from build123d import *

# Parameters (mm, degrees)
BOSS_EXTRUDE1_DEPTH      = 50
BOSS_EXTRUDE1_DEPTH_BACK = 50
SKETCH2_W                = 10
SKETCH2_H                = 3
SKETCH3_W                = 5
SKETCH3_H                = 3
SKETCH5_R                = 1.5
CUT_EXTRUDE2_DEPTH       = 3


with BuildPart() as part:
    # Sketch2 → Boss-Extrude1 (new, two sides: drawn at the far end of the back side and taken through both)
    with BuildSketch(Plane.XY.offset(-BOSS_EXTRUDE1_DEPTH_BACK)):
        with Locations((-5, -1)):
            Rectangle(SKETCH2_W, SKETCH2_H)
    extrude(amount=BOSS_EXTRUDE1_DEPTH + BOSS_EXTRUDE1_DEPTH_BACK)

    # Sketch3 → Revolve1 (revolve)
    with BuildSketch(Plane.XY.offset(50)):
        with Locations((-2.5, -1)):
            Rectangle(SKETCH3_W, SKETCH3_H)
    revolve1 = revolve(axis=Axis((-5, 0.5, 50), (0, -1, 0)))

    # Mirror1: Revolve1 across plane
    add(revolve1.mirror(Plane.XY))

    # Sketch5 → Cut-Extrude2 (cut)
    with BuildSketch(Plane(origin=(0, -2.5, 0), x_dir=(-1, 0, 0), z_dir=(0, -1, 0))):
        with Locations(Location((5, -50, 0), (0, 0, 180))):
            Circle(SKETCH5_R)
    cut_extrude2 = extrude(amount=-CUT_EXTRUDE2_DEPTH, mode=Mode.SUBTRACT)

    # Mirror2: Cut-Extrude2 across plane
    add(cut_extrude2.mirror(Plane.XY), mode=Mode.SUBTRACT)


solid = part.part
Input: part model. Units: mm. Frame: model coordinates. Round coordinates to 2 decimals unless told otherwise and drop trailing zeros. Write each loop counter-clockwise with the first axis right and the second up, starting at its lowest first coordinate (ties: lowest second). Pieces come first, ordered by that corner, then holes.
1) Contact query for a flat-ended pin moving along its axis: P1, Ø1, axis at x = -8.5, y = -1.5, coming from the +Z side. Output: stop coordinate, or through.
2) Ray query, L1, parallel to Z at x = -5, y = -0.65; L2, parallel to X at y = -0.55, z = -50; L3, parallel to Z at x = -4.5, y = -2.25. Return the intervals inside material, ascending.
3) Cut plane B-B (y = -2). Return the cut outline in (x, z).
4) Draft query along X for faces 1 (the cylindrical face through (-5.325, -1.021, -48.536)), 2 (the flat face through (-5, 0.5, -1)), 3 (the cylindrical face through (-5, -1, 55)), 4 (the cylindrical face through (-5.325, -1.021, 48.536)). Return one class per face: pulls with the +X half, pulls with the -X half, needs draft (parallel to the pull), parting line crosses it, or undercut.
5) Cut plane A-A (x = -5). Return the cut outline in (y, z), then the cut area to 3 significant figures.
Geometry says:
1. P1: stops at z = 54
2. L1: z = -55 to -51.5, -48.5 to 48.5, 51.5 to 55
2. L2: x = -10 to -6.5, -3.5 to 0
2. L3: z = -54.97 to -51.41, -48.59 to 48.59, 51.41 to 54.97
3. outline: (-10, -50) arc R5 ccw to (0, -50) - (0, 50) arc R5 ccw to (-10, 50) - close; hole circle Ø3 at (-5, -50); hole circle Ø3 at (-5, 50)
4. face 1: undercut
4. face 2: needs draft
4. face 3: parting line crosses it
4. face 4: undercut
5. outline: (-2.5, -55) - (0.5, -55) - (0.5, -51.5) - (-2.5, -51.5) - close; (-2.5, -48.5) - (0.5, -48.5) - (0.5, 48.5) - (-2.5, 48.5) - close; (-2.5, 51.5) - (0.5, 51.5) - (0.5, 55) - (-2.5, 55) - close
5. area: 312 mm2
